from build123d import *

# Parameters (mm, degrees)
MODEL_R             = 2.5
BOSS_EXTRUDE1_DEPTH = 4
SKETCH2_R           = 2.95
CUT_EXTRUDE1_DEPTH  = 4
SKETCH3_R           = 1.35
CUT_EXTRUDE2_DEPTH  = 4
CIRPATTERN1_COUNT   = 3
BOSS_EXTRUDE2_DEPTH = 4


with BuildPart() as part:
    # Model → Boss-Extrude1 (new body)
    with BuildSketch(Plane.XY):
        with BuildLine():
            ThreePointArc((-11.997000624, 0.268283487), (-12, 0), (-11.997000624, -0.268283487))
            ThreePointArc((-11.997000624, -0.268283487), (-10.895606779, -0.741380557), (-9.707399683, -0.89966238))
            ThreePointArc((-9.707399683, -0.89966238), (-9.649769237, -1.387427358), (-9.56764597, -1.8716708))
            ThreePointArc((-9.56764597, -1.8716708), (-10.663129188, -2.358297721), (-11.586621996, -3.122529539))
            ThreePointArc((-11.586621996, -3.122529539), (-11.513915683, -3.380790682), (-11.43545361, -3.637361781))
            ThreePointArc((-11.43545361, -3.637361781), (-10.245387108, -3.780996591), (-9.060717605, -3.598110265))
            ThreePointArc((-9.060717605, -3.598110265), (-8.868002323, -4.049880962), (-8.652778483, -4.491372344))
            ThreePointArc((-8.652778483, -4.491372344), (-9.566788286, -5.266920743), (-10.237564162, -6.260373793))
            ThreePointArc((-10.237564162, -6.260373793), (-10.095042394, -6.487689809), (-9.947474154, -6.711762656))
            ThreePointArc((-9.947474154, -6.711762656), (-8.765147105, -6.514298768), (-7.679990073, -6.005060656))
            ThreePointArc((-7.679990073, -6.005060656), (-7.3678026, -6.384237295), (-7.036914342, -6.747209612))
            ThreePointArc((-7.036914342, -6.747209612), (-7.695403093, -7.74884917), (-8.059119765, -8.891039794))
            ThreePointArc((-8.059119765, -8.891039794), (-7.858328807, -9.068994892), (-7.653609502, -9.242416436))
            ThreePointArc((-7.653609502, -9.242416436), (-6.574807012, -8.719851201), (-5.67707542, -7.925516745))
            ThreePointArc((-5.67707542, -7.925516745), (-5.270707329, -8.201380692), (-4.850961252, -8.456428084))
            ThreePointArc((-4.850961252, -8.456428084), (-5.200582107, -9.603011921), (-5.227773414, -10.801406627))
            ThreePointArc((-5.227773414, -10.801406627), (-4.984980156, -10.915583944), (-4.739694926, -11.024304604))
            ThreePointArc((-4.739694926, -11.024304604), (-3.851815156, -10.218973149), (-3.214237879, -9.203894603))
            ThreePointArc((-3.214237879, -9.203894603), (-2.746610697, -9.354097), (-2.27201213, -9.480557045))
            ThreePointArc((-2.27201213, -9.480557045), (-2.284440889, -10.679195758), (-1.972903952, -11.836707735))
            ThreePointArc((-1.972903952, -11.836707735), (-1.707778059, -11.877857303), (-1.441798455, -11.913069177))
            ThreePointArc((-1.441798455, -11.913069177), (-0.816772145, -10.890214666), (-0.491001901, -9.736627657))
            ThreePointArc((-0.491001901, -9.736627657), (0, -9.749), (0.491001901, -9.736627657))
            ThreePointArc((0.491001901, -9.736627657), (0.816772145, -10.890214666), (1.441798455, -11.913069177))
            ThreePointArc((1.441798455, -11.913069177), (1.707778059, -11.877857303), (1.972903952, -11.836707735))
            ThreePointArc((1.972903952, -11.836707735), (2.284440889, -10.679195758), (2.27201213, -9.480557045))
            ThreePointArc((2.27201213, -9.480557045), (2.746610697, -9.354097), (3.214237879, -9.203894603))
            ThreePointArc((3.214237879, -9.203894603), (3.851815156, -10.218973149), (4.739694926, -11.024304604))
            ThreePointArc((4.739694926, -11.024304604), (4.984980156, -10.915583944), (5.227773414, -10.801406627))
            ThreePointArc((5.227773414, -10.801406627), (5.200582107, -9.603011921), (4.850961252, -8.456428084))
            ThreePointArc((4.850961252, -8.456428084), (5.270707329, -8.201380692), (5.67707542, -7.925516745))
            ThreePointArc((5.67707542, -7.925516745), (6.574807012, -8.719851201), (7.653609502, -9.242416436))
            ThreePointArc((7.653609502, -9.242416436), (7.858328807, -9.068994892), (8.059119765, -8.891039794))
            ThreePointArc((8.059119765, -8.891039794), (7.695403093, -7.74884917), (7.036914342, -6.747209612))
            ThreePointArc((7.036914342, -6.747209612), (7.3678026, -6.384237295), (7.679990073, -6.005060656))
            ThreePointArc((7.679990073, -6.005060656), (8.765147105, -6.514298768), (9.947474154, -6.711762656))
            ThreePointArc((9.947474154, -6.711762656), (10.095042394, -6.487689809), (10.237564162, -6.260373793))
            ThreePointArc((10.237564162, -6.260373793), (9.566788286, -5.266920743), (8.652778482, -4.491372344))
            ThreePointArc((8.652778482, -4.491372344), (8.868002323, -4.049880962), (9.060717605, -3.598110265))
            ThreePointArc((9.060717605, -3.598110265), (10.245387108, -3.780996591), (11.43545361, -3.637361781))
            ThreePointArc((11.43545361, -3.637361781), (11.513915683, -3.380790682), (11.586621996, -3.122529539))
            ThreePointArc((11.586621996, -3.122529539), (10.663129188, -2.358297721), (9.56764597, -1.8716708))
            ThreePointArc((9.56764597, -1.8716708), (9.649769237, -1.387427358), (9.707399683, -0.89966238))
            ThreePointArc((9.707399683, -0.89966238), (10.895606779, -0.741380557), (11.997000624, -0.268283487))
            ThreePointArc((11.997000624, -0.268283487), (12, 0), (11.997000624, 0.268283487))
            ThreePointArc((11.997000624, 0.268283487), (10.895606779, 0.741380557), (9.707399683, 0.89966238))
            ThreePointArc((9.707399683, 0.89966238), (9.649769237, 1.387427358), (9.56764597, 1.8716708))
            ThreePointArc((9.56764597, 1.8716708), (10.663129188, 2.358297721), (11.586621996, 3.122529539))
            ThreePointArc((11.586621996, 3.122529539), (11.513915683, 3.380790682), (11.43545361, 3.637361781))
            ThreePointArc((11.43545361, 3.637361781), (10.245387108, 3.780996591), (9.060717605, 3.598110265))
            ThreePointArc((9.060717605, 3.598110265), (8.868002323, 4.049880962), (8.652778483, 4.491372344))
            ThreePointArc((8.652778483, 4.491372344), (9.566788286, 5.266920743), (10.237564162, 6.260373793))
            ThreePointArc((10.237564162, 6.260373793), (10.095042394, 6.487689809), (9.947474154, 6.711762656))
            ThreePointArc((9.947474154, 6.711762656), (8.765147105, 6.514298768), (7.679990073, 6.005060656))
            ThreePointArc((7.679990073, 6.005060656), (7.3678026, 6.384237295), (7.036914342, 6.747209612))
            ThreePointArc((7.036914342, 6.747209612), (7.695403093, 7.74884917), (8.059119765, 8.891039794))
            ThreePointArc((8.059119765, 8.891039794), (7.858328807, 9.068994892), (7.653609502, 9.242416436))
            ThreePointArc((7.653609502, 9.242416436), (6.574807012, 8.719851201), (5.67707542, 7.925516745))
            ThreePointArc((5.67707542, 7.925516745), (5.270707329, 8.201380692), (4.850961252, 8.456428084))
            ThreePointArc((4.850961252, 8.456428084), (5.200582107, 9.603011921), (5.227773414, 10.801406627))
            ThreePointArc((5.227773414, 10.801406627), (4.984980156, 10.915583944), (4.739694926, 11.024304604))
            ThreePointArc((4.739694926, 11.024304604), (3.851815156, 10.218973149), (3.214237879, 9.203894603))
            ThreePointArc((3.214237879, 9.203894603), (2.746610697, 9.354097), (2.27201213, 9.480557045))
            ThreePointArc((2.27201213, 9.480557045), (2.284440889, 10.679195758), (1.972903952, 11.836707735))
            ThreePointArc((1.972903952, 11.836707735), (1.707778059, 11.877857303), (1.441798455, 11.913069177))
            ThreePointArc((1.441798455, 11.913069177), (0.816772145, 10.890214666), (0.491001901, 9.736627657))
            ThreePointArc((0.491001901, 9.736627657), (0, 9.749), (-0.491001901, 9.736627657))
            ThreePointArc((-0.491001901, 9.736627657), (-0.816772145, 10.890214666), (-1.441798455, 11.913069177))
            ThreePointArc((-1.441798455, 11.913069177), (-1.707778059, 11.877857303), (-1.972903952, 11.836707735))
            ThreePointArc((-1.972903952, 11.836707735), (-2.284440889, 10.679195758), (-2.27201213, 9.480557045))
            ThreePointArc((-2.27201213, 9.480557045), (-2.746610697, 9.354097), (-3.214237879, 9.203894603))
            ThreePointArc((-3.214237879, 9.203894603), (-3.851815156, 10.218973149), (-4.739694926, 11.024304604))
            ThreePointArc((-4.739694926, 11.024304604), (-4.984980156, 10.915583944), (-5.227773414, 10.801406627))
            ThreePointArc((-5.227773414, 10.801406627), (-5.200582107, 9.603011921), (-4.850961252, 8.456428084))
            ThreePointArc((-4.850961252, 8.456428084), (-5.270707329, 8.201380692), (-5.67707542, 7.925516745))
            ThreePointArc((-5.67707542, 7.925516745), (-6.574807012, 8.719851201), (-7.653609502, 9.242416436))
            ThreePointArc((-7.653609502, 9.242416436), (-7.858328807, 9.068994892), (-8.059119765, 8.891039794))
            ThreePointArc((-8.059119765, 8.891039794), (-7.695403093, 7.74884917), (-7.036914342, 6.747209612))
            ThreePointArc((-7.036914342, 6.747209612), (-7.3678026, 6.384237295), (-7.679990073, 6.005060656))
            ThreePointArc((-7.679990073, 6.005060656), (-8.765147105, 6.514298768), (-9.947474154, 6.711762656))
            ThreePointArc((-9.947474154, 6.711762656), (-10.095042394, 6.487689809), (-10.237564162, 6.260373793))
            ThreePointArc((-10.237564162, 6.260373793), (-9.566788286, 5.266920743), (-8.652778482, 4.491372344))
            ThreePointArc((-8.652778482, 4.491372344), (-8.868002323, 4.049880962), (-9.060717605, 3.598110265))
            ThreePointArc((-9.060717605, 3.598110265), (-10.245387108, 3.780996591), (-11.43545361, 3.637361781))
            ThreePointArc((-11.43545361, 3.637361781), (-11.513915683, 3.380790682), (-11.586621996, 3.122529539))
            ThreePointArc((-11.586621996, 3.122529539), (-10.663129188, 2.358297721), (-9.56764597, 1.8716708))
            ThreePointArc((-9.56764597, 1.8716708), (-9.649769237, 1.387427358), (-9.707399683, 0.89966238))
            ThreePointArc((-9.707399683, 0.89966238), (-10.895606779, 0.741380557), (-11.997000624, 0.268283487))
        make_face()
        Circle(MODEL_R, mode=Mode.SUBTRACT)
    extrude(amount=BOSS_EXTRUDE1_DEPTH)

    # Sketch2 → Cut-Extrude1 (cut)
    with BuildSketch(Plane.XY.offset(4)):
        Circle(SKETCH2_R)
    extrude(amount=-CUT_EXTRUDE1_DEPTH, mode=Mode.SUBTRACT)

    # Sketch3 → Cut-Extrude2 (cut)
    with BuildSketch(Plane.XY.offset(4)):
        with Locations((-6, 0)):
            Circle(SKETCH3_R)
    cut_extrude2 = extrude(amount=-CUT_EXTRUDE2_DEPTH, mode=Mode.SUBTRACT)

    # CirPattern1: Cut-Extrude2 ×3 about axis
    cirpattern1_axis = Axis((0, 0, 0), (0, 0, 1))
    for i in range(1, CIRPATTERN1_COUNT):
        add(cut_extrude2.rotate(cirpattern1_axis, i * 360 / CIRPATTERN1_COUNT), mode=Mode.SUBTRACT)

    # Sketch5 → Boss-Extrude2 (add)
    with BuildSketch(Plane.XY):
        with BuildLine():
            ThreePointArc((-2.95, 0), (-2.941926879, -0.218096855), (-2.917751703, -0.435))
            Line((-2.917751703, -0.435), (2.917751703, -0.435))
            ThreePointArc((2.917751703, -0.435), (2.941926879, -0.218096855), (2.95, 0))
            ThreePointArc((2.95, 0), (2.941926879, 0.218096855), (2.917751703, 0.435))
            Line((2.917751703, 0.435), (-2.917751703, 0.435))
            ThreePointArc((-2.917751703, 0.435), (-2.941926879, 0.218096855), (-2.95, 0))
        make_face()
    extrude(amount=BOSS_EXTRUDE2_DEPTH)


solid = part.part
Could you check a few things on this model? Use its own coordinates, in mm. A direction names the side the tool comes from. Give positions to 0.01 mm unless a question says otherwise; leave off trailing zeros. Loops run counter-clockwise (first coordinate to the right, second up) from the corner with the lowest first, then second, coordinate; pieces in that order, holes last. Notation, with made-up numbers: M 68,64 L 111,64 A18 ccw 111,98 Z; hole C -8,14.25 d1. An arc over 180 degrees is marked long. Answer as a JSON object with one key per item and string values.
Q1. If we mould it in two halves opening along Y, with no side actions, what happens to faces 5 (the cylindrical face through (8.75, -6.51, 1.97)), 6 (the cylindrical face through (6.59, 8.73, 1.97))? For each: pulls with the +Y half, pulls with the -Y half, needs draft (parallel to the pull), parting line crosses it, or undercut.
Values found:
{"face 5": "undercut", "face 6": "pulls with the +Y half"}
Q2. For P1, Ø1, axis at x = -1.5, z = 0.5, coming from the -Y side; P2, Ø2, axis at x = -2.5, z = 2, coming from the +Y side, each with a flat end and sliding along its axis, tell me the tip position at first contact or that it passes through.
Values found:
{"P1": "stops at y = -11.91", "P2": "stops at y = 11.91"}
Q3. Suppose I cut it at A-A, the plane x = 3.5. List the corners of the cut face in (y, z) for me, plus the area to 3 significant figures.
Values found:
{"outline": "M -9.74,0 L -6.45,0 L -6.45,4 L -9.74,4 Z; M -3.94,0 L 3.94,0 L 3.94,4 L -3.94,4 Z; M 6.45,0 L 9.74,0 L 9.74,4 L 6.45,4 Z", "area": "57.8 mm²"}
Q4. Suppose I cut it at B-B, the plane x = -6. List the corners of the cut face in (y, z) for me, plus the area to 3 significant figures.
Values found:
{"outline": "M -8.26,0 L -1.35,0 L -1.35,4 L -8.26,4 Z; M 1.35,0 L 8.26,0 L 8.26,4 L 1.35,4 Z", "area": "55.3 mm²"}
Q5. Suppose I cut it at C-C, the plane x = -1. List the corners of the cut face in (y, z) for me (3 decimals), plus the area to 3 significant figures.
Values found:
{"outline": "M -11.261,0 L -2.775,0 L -2.775,4 L -11.261,4 Z; M -0.435,0 L 0.435,0 L 0.435,4 L -0.435,4 Z; M 2.775,0 L 11.261,0 L 11.261,4 L 2.775,4 Z", "area": "71.4 mm²"}
Q6. For faces 1 (the cylindrical face through (9.58, -5.28, 1.97)), 2 (the cylindrical face through (5.26, -8.21, 1.97)), 3 (the cylindrical face through (-3.841, 10.206, 1.972)), 4 (the cylindrical face through (-7.688, -7.734, 1.972)), which set-ups out of +Z, -Z, +X, -X, +Y, -Y let a thin tool reach every point of the face, with its end or its side?
Values found:
{"face 1": "+Z, -Z, +X", "face 2": "+Z, -Z", "face 3": "+Z, -Z, +Y", "face 4": "+Z, -Z, -X"}
Q7. If I drill on probe 1 along Y at (x, z) = (1, 1.6) (3 decimals); probe 2 along Y at (x, z) = (-7.75, 3.45); probe 3 along X at (y, z) = (-0.5, 2.2), over which ranges is the centre line in solid material (lowest first)? Write a range as [from, to].
Values found:
{"probe 1": "y = [-11.261, -2.775], [-0.435, 0.435], [2.775, 11.261]", "probe 2": "y = [-9.16, -7.87], [-6.05, 6.05], [7.87, 9.16]", "probe 3": "x = [-11.56, -7.25], [-4.75, -2.91], [2.91, 11.56]"}
